The model under review builds one solid part; all positions refer to its coordinate system, in mm. Face numbers are marked on the shaded views. Coordinates: 2 decimals unless noted, no trailing zeros. Write each loop counter-clockwise with the first axis right and the second up, starting at its lowest first coordinate (ties: lowest second). Pieces come first, ordered by that corner, then holes.
1) For P1, Ø5.5, axis at y = 0, z = 0, coming from the -X side; P2, Ø5, axis at x = 31, z = -3, coming from the +Y side; P3, Ø1, axis at x = 8.5, y = -3, coming from the -Z side; P4, Ø5, axis at x = 37.5, y = 2, coming from the +Z side, all flat-tipped, find the tip position at first contact; note any pin that passes through.
2) Add section B-B, the plane x = 18. State the section outline as (y, z) points, then the cut area to 3 significant figures.
3) For line 1 (Z direction, x = 8.5, y = 0.25); line 2 (Y direction, x = 11, z = 0); line 3 (Y direction, x = 3.5, z = -2.5), list the stretches that pass through material, from the lowest coordinate up.
4) Mouldability with a two-part tool opening along Z and no side actions: class the marked faces 1 and 2 as released by +Z, released by -Z, zero draft, split by the parting line, or undercut.
5) Add section A-A, the plane x = 30.5. State the section outline as (y, z) points.
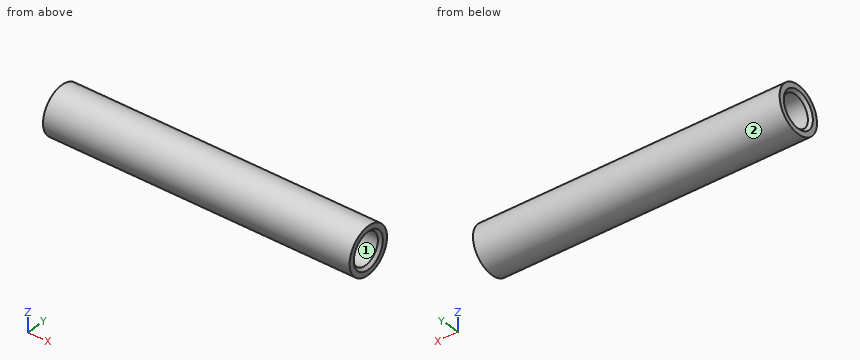
from build123d import *

# Parameters (mm, degrees)
SKETCH_1_R                      = 5
EXTRUDE_2_DEPTH                 = 65
HOLE_WIZARD_G1_16_1_D           = 6.6
HOLE_WIZARD_G1_16_1_DEPTH       = 20
HOLE_WIZARD_G1_16_1_CSINK_D     = 7.773
HOLE_WIZARD_G1_16_1_CSINK_ANGLE = 90
HOLE_WIZARD_G1_16_1_TIP         = 1.982840043
HOLE_WIZARD_G1_16_2_D           = 6.6
HOLE_WIZARD_G1_16_2_DEPTH       = 20
HOLE_WIZARD_G1_16_2_CSINK_D     = 7.773
HOLE_WIZARD_G1_16_2_CSINK_ANGLE = 90
HOLE_WIZARD_G1_16_2_TIP         = 1.982840043


with BuildPart() as part:
    # 草图1 → 凸台-拉伸2 (new body)
    with BuildSketch(Plane(origin=(0, 0, 0), x_dir=(0, 0, -1), z_dir=(1, 0, 0))):
        Circle(SKETCH_1_R)
    extrude(amount=EXTRUDE_2_DEPTH)

    # G1/16 螺纹孔1
    with Locations(Plane.ZY):
        with Locations((0, 0)):
            CounterSinkHole(HOLE_WIZARD_G1_16_1_D / 2, HOLE_WIZARD_G1_16_1_CSINK_D / 2, depth=HOLE_WIZARD_G1_16_1_DEPTH, counter_sink_angle=HOLE_WIZARD_G1_16_1_CSINK_ANGLE)
            with Locations((0, 0, -(HOLE_WIZARD_G1_16_1_DEPTH + HOLE_WIZARD_G1_16_1_TIP / 2))):  # 118° drill point
                Cone(0, HOLE_WIZARD_G1_16_1_D / 2, HOLE_WIZARD_G1_16_1_TIP, mode=Mode.SUBTRACT)

    # G1/16 螺纹孔2
    with Locations(Plane(origin=(65, 0, 0), x_dir=(0, 0, -1), z_dir=(1, 0, 0))):
        with Locations((0, 0)):
            CounterSinkHole(HOLE_WIZARD_G1_16_2_D / 2, HOLE_WIZARD_G1_16_2_CSINK_D / 2, depth=HOLE_WIZARD_G1_16_2_DEPTH, counter_sink_angle=HOLE_WIZARD_G1_16_2_CSINK_ANGLE)
            with Locations((0, 0, -(HOLE_WIZARD_G1_16_2_DEPTH + HOLE_WIZARD_G1_16_2_TIP / 2))):  # 118° drill point
                Cone(0, HOLE_WIZARD_G1_16_2_D / 2, HOLE_WIZARD_G1_16_2_TIP, mode=Mode.SUBTRACT)


solid = part.part
Geometry results:
1. P1: stops at x = 20.33
1. P2: stops at y = 4.97
1. P3: stops at z = -4.33
1. P4: stops at z = 5
2. outline: circle Ø10 at (0, 0); hole circle Ø6.6 at (0, 0)
2. area: 44.3 mm2
3. line 1: z = -4.99 to -3.29, 3.29 to 4.99
3. line 2: y = -5 to -3.3, 3.3 to 5
3. line 3: y = -4.33 to -2.15, 2.15 to 4.33
4. face 1: undercut
4. face 2: split by the parting line
5. outline: circle Ø10 at (0, 0)
